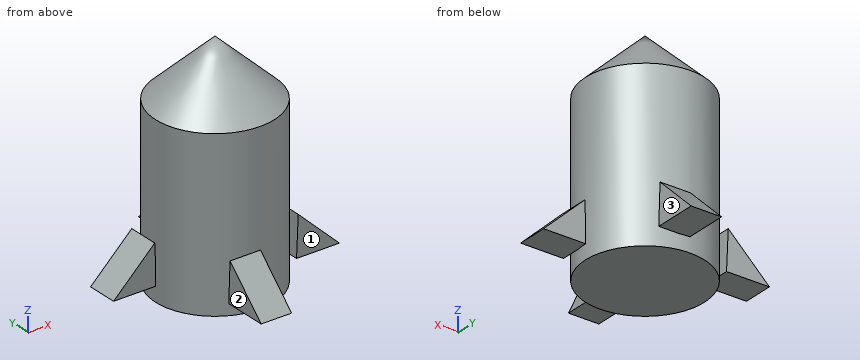
```python
from build123d import *

# Parameters (mm, degrees)
F3_DEPTH        = 10
F3_COPIES_COUNT = 4


# Not quite as in the source:
# - a pattern or mirror of a feature is missing from the dataset's text; its kind, count and spacing are read off the source's solid


with BuildPart() as f1:
    # F0 (on Front) → F1 (revolve)
    with BuildSketch(Plane.XZ):
        Polygon((19.5114035159, 23.0333190411), (0, 41.6290275753), (0, -31.3450358808), (19.5114035159, -31.3450358808), align=None)
    revolve(axis=Axis((0, 0, 5.1419958472), (0, 0, -1)))

    # F2 (on Right) → F3 (join)
    with BuildSketch(Plane.YZ):
        Polygon((-19.2296542227, -26.5552345663), (-19.7931565344, -13.5945891961), (-33.3173125982, -26.5552345663), align=None)
    f3 = extrude(amount=-F3_DEPTH)

    # F3_copies: F3 ×4 about axis
    f3_copies_axis = Axis((0, 0, 0), (0, 0, 1))
    for i in range(1, F3_COPIES_COUNT):
        add(f3.rotate(f3_copies_axis, i * 360 / F3_COPIES_COUNT))


solid = f1.part
```
Could you check a few things on this model? Use its own coordinates, in mm. Face numbers are marked on the shaded views. A direction names the side the tool comes from. Coordinates: 2 decimals unless noted, no trailing zeros. Write each loop counter-clockwise with the first axis right and the second up, starting at its lowest first coordinate (ties: lowest second). Pieces come first, ordered by that corner, then holes. Notation, with made-up numbers: (83, 26) -> (126, 26) arc R22 cw to (126, 62) -> close; hole circle Ø10 at (74.5, -31.5). An arc over 180 degrees is marked (long way). Return JSON: item names as keys, results as strings.
(1) Imagine slicing it at A-A, the plane y = 21. Please give me the cut outline in (x, z).
Numbers:
{"outline": "(0, -26.56) -> (10, -26.56) -> (10, -14.75) -> (0, -14.75) -> close"}
(2) Imagine slicing it at D-D, the plane y = -27.5. Please give me the cut outline in (x, z).
Numbers:
{"outline": "(-10, -26.56) -> (0, -26.56) -> (0, -20.98) -> (-10, -20.98) -> close"}
(3) Imagine slicing it at C-C, the plane z = 35. Please give me the cut outline in (x, y), then the cut area to 3 significant figures.
Numbers:
{"outline": "circle Ø13.91 at (0, 0)", "area": "152 mm2"}
(4) Which directions (+Z, -Z, +X, -X, +Y, -Y) give clear straight access to the entire face, cutting with the end or side of a thin tool? Please do the marked faces 1, 2 and 3.
Numbers:
{"face 1": "+Z, -Z, +X, -Y", "face 2": "+Z, -Z, -X, -Y", "face 3": "+Z, -Z, +X, +Y"}
(5) Imagine slicing it at B-B, the plane z = 25.5. Please give me the cut outline in (x, y).
Numbers:
{"outline": "circle Ø33.85 at (0, 0)"}
(6) I'm going to push flat-ended pins straight in: pin 1 (3 mm diameter, centred on y = 10.5, z = -8, fed in from +X); pin 2 (14.5 mm diameter, centred on x = -28, z = -23, fed in from +Y); pin 3 (8 mm diameter, centred on x = 28.5, y = -7, fed in from -Z). Where does each tip first touch, or does it pass through?
Numbers:
{"pin 1": "stops at x = 17.31", "pin 2": "stops at y = 10", "pin 3": "stops at z = -26.56"}
(7) I need wall thicknesses on L1, parallel to X at y = -0.5, z = -15 (3 decimals); L2, parallel to X at y = 0.5, z = 11 (3 decimals); L3, parallel to Y at x = 2, z = 33.5. Which ranges of each line are inside material? Lowest first, please.
Numbers:
{"L1": "x = -19.505 to 19.505, 19.732 to 21.26", "L2": "x = -19.505 to 19.505", "L3": "y = -8.29 to 8.29"}
